Geometry check sheet. Reference: drawing and pictorial views, mm from the part's lowest x, y, z. A direction names the side the tool comes from. Give positions to 0.01 mm unless a question says otherwise; leave off trailing zeros. Order: outer loops, then holes, each group sorted by start corner. A loop starts at its lowest first (then second) coordinate and runs counter-clockwise, first axis right, second up. Notation, with made-up numbers: M 77,60.5 L 111,60.5 A8 cw 111,70.5 Z; hole C 34.5,11 d7. An arc over 180 degrees is marked long. Answer as CSV lines item,"result".
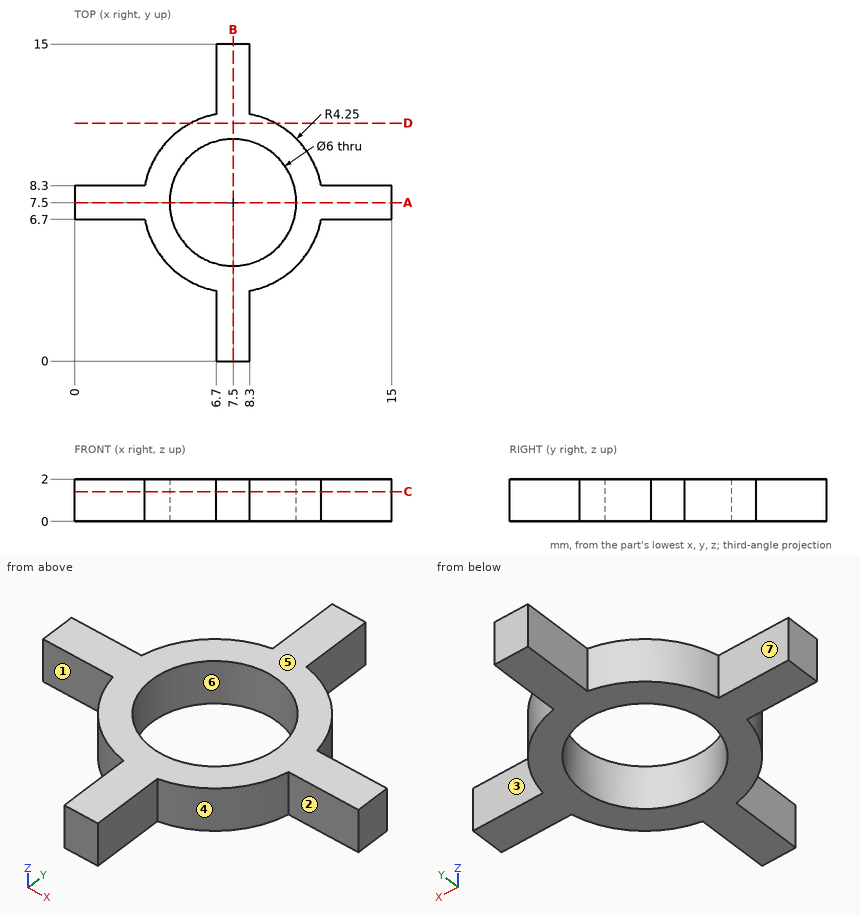
(1) Gauge pin test, flat ends, axial feed: P1, Ø5, axis at x = 7.5, y = 7.5, coming from the -Z side; P2, Ø1, axis at y = 2, z = 1.5, coming from the +X side; P3, Ø0.6, axis at x = 2, z = 1, coming from the +Y side; P4, Ø1, axis at x = 13, z = 1, coming from the -Y side. Record the tip position at first contact, or that the pin passes through.
The answers:
P1,"passes through"
P2,"stops at x = 8.3"
P3,"stops at y = 8.3"
P4,"stops at y = 6.7"
(2) Section check C-C on z = 1.4. Enter the section's corners in (x, y), then the cut area to 3 significant figures.
The answers:
outline,"M 0,6.7 L 3.33,6.7 A4.25 ccw 6.7,3.33 L 6.7,0 L 8.3,0 L 8.3,3.33 A4.25 ccw 11.67,6.7 L 15,6.7 L 15,8.3 L 11.67,8.3 A4.25 ccw 8.3,11.67 L 8.3,15 L 6.7,15 L 6.7,11.67 A4.25 ccw 3.33,8.3 L 0,8.3 Z; hole C 7.5,7.5 d6"
area,"49.4 mm2"
(3) Tool access check on the marked faces 1, 2 and 3. Record the directions out of +Z, -Z, +X, -X, +Y, -Y that give a thin tool (end or side, any length) a straight path to the whole face; none if there is none.
The answers:
face 1,"+Z, -Z, -X, -Y"
face 2,"+Z, -Z, +X, -Y"
face 3,"+Z, -Z, +X, +Y"
(4) Section check D-D on y = 11.25. Enter the section's corners in (x, z), then the cut area to 3 significant figures.
The answers:
outline,"M 5.5,0 L 9.5,0 L 9.5,2 L 5.5,2 Z"
area,"8.00 mm2"
(5) Draft check along Y on the marked faces 4, 5, 6 and 7. Enter one of: +Y half, -Y half, draft (parallel to the pull), parting line (faces both ways), or undercut.
The answers:
face 4,"-Y half"
face 5,"draft"
face 6,"undercut"
face 7,"+Y half"
(6) Section check A-A on y = 7.5. Enter the section's corners in (x, z).
The answers:
outline,"M 0,0 L 4.5,0 L 4.5,2 L 0,2 Z; M 10.5,0 L 15,0 L 15,2 L 10.5,2 Z"
(7) Material ranges on line 1 (Y direction, x = 7.5, z = 1.5); line 2 (Y direction, x = 10, z = 1.6); line 3 (X direction, y = 7, z = 1.8), recorded low to high.
The answers:
line 1,"y = 0 to 4.5, 10.5 to 15"
line 2,"y = 4.06 to 5.84, 9.16 to 10.94"
line 3,"x = 0 to 4.54, 10.46 to 15"
